from build123d import *

# Parameters (mm, degrees)
F0_W     = 101.6
F0_H     = 101.6
F0_W_2   = 88.9
F0_H_2   = 88.9
F1_DEPTH = 914.4
F2_R     = 6.35


with BuildPart() as f1:
    # F0 (on Front) → F1 (new body, symmetric)
    with BuildSketch(Plane.XZ):
        Rectangle(F0_W, F0_H)
        Rectangle(F0_W_2, F0_H_2, mode=Mode.SUBTRACT)
    extrude(amount=F1_DEPTH, both=True)

    # F2
    f2_edges = [f1.edges().sort_by_distance(p)[0] for p in [
        (-50.8, 0, 50.8),
        (50.8, 0, 50.8),
        (44.45, 0, -44.45),
        (-44.45, 0, -44.45),
        (44.45, 0, 44.45),
        (-44.45, 0, 44.45),
        (50.8, 0, -50.8),
        (-50.8, 0, -50.8),
    ]]
    fillet(f2_edges, radius=F2_R)


solid = f1.part
Model file for the job. Use its own axes, mm. A direction names the side the tool comes from. Give positions to 0.01 mm unless a question says otherwise; leave off trailing zeros. Loops run counter-clockwise (first coordinate to the right, second up) from the corner with the lowest first, then second, coordinate; pieces in that order, holes last. Notation, with made-up numbers: (32.25, 71) -> (41.25, 71) arc R25 cw to (41.25, 103) -> close; hole circle Ø2 at (4.5, 36.25). An arc over 180 degrees is marked (long way). Use a Markdown table: item, result. Add a question column.
(1) Slice it at B-B on z = 4. List the corners of the cut face in (x, y), and give its area (3 significant figures).
(2) Mould opens along X. For faces 1 (the flat face through (4, -914.4, -45)), 2 (the flat face through (44.45, -13, -1)), 3 (the flat face through (-1, -13, -44.45)), 4 (the flat face through (-50.8, -13, -1)) say: +X half, -X half, draft (parallel to the pull), parting line (faces both ways), or undercut.
(3) Slice it at C-C on y = -159.5. List the corners of the cut face in (x, z), and give its area (3 significant figures).
(4) Slice it at A-A on x = 3. List the corners of the cut face in (y, z).
(5) Tool access for faces 5 (the flat face through (-1, -13, 44.45)), 6 (the flat face through (-1, -13, -50.8)): list every direction of +Z, -Z, +X, -X, +Y, -Y with a clear straight run to the whole face (end or side of a thin tool).
(6) Wall check: line 1 along Z through (x, y) = (25, -764.5); line 2 along Z through (x, y) = (-43, -814.5). Give the ranges that are in metal, low to high.
Filled sheet:
| question | item | result |
|---|---|---|
| 1 | outline | (-50.8, -914.4) -> (-44.45, -914.4) -> (-44.45, 914.4) -> (-50.8, 914.4) -> close; (44.45, -914.4) -> (50.8, -914.4) -> (50.8, 914.4) -> (44.45, 914.4) -> close |
| 1 | area | 23,200 mm2 |
| 2 | face 1 | draft |
| 2 | face 2 | undercut |
| 2 | face 3 | undercut |
| 2 | face 4 | -X half |
| 3 | outline | (-50.8, -44.45) arc R6.35 ccw to (-44.45, -50.8) -> (44.45, -50.8) arc R6.35 ccw to (50.8, -44.45) -> (50.8, 44.45) arc R6.35 ccw to (44.45, 50.8) -> (-44.45, 50.8) arc R6.35 ccw to (-50.8, 44.45) -> close; hole (-44.45, -38.1) arc R6.35 ccw to (-38.1, -44.45) -> (38.1, -44.45) arc R6.35 ccw to (44.45, -38.1) -> (44.45, 38.1) arc R6.35 ccw to (38.1, 44.45) -> (-38.1, 44.45) arc R6.35 ccw to (-44.45, 38.1) -> close |
| 3 | area | 2,420 mm2 |
| 4 | outline | (-914.4, -50.8) -> (914.4, -50.8) -> (914.4, -44.45) -> (-914.4, -44.45) -> close; (-914.4, 44.45) -> (914.4, 44.45) -> (914.4, 50.8) -> (-914.4, 50.8) -> close |
| 5 | face 5 | +Y, -Y |
| 5 | face 6 | -Z, +X, -X, +Y, -Y |
| 6 | line 1 | -50.8 to -44.45, 44.45 to 50.8 |
| 6 | line 2 | -50.8 to -42.14, 42.14 to 50.8 |
